```python
from build123d import *

# Parameters (mm, degrees)
SKETCH1_R                = 2
SKETCH1_R_2              = 2.5
BOSS_EXTRUDE1_DEPTH      = 5
BOSS_EXTRUDE2_DEPTH      = 6.5
BOSS_EXTRUDE2_DEPTH_BACK = 1.5
SKETCH2_R                = 2
CUT_EXTRUDE1_DEPTH       = 100
FILLET1_R                = 0.5


with BuildPart() as part:
    # Sketch1 → Boss-Extrude1 (new body)
    with BuildSketch(Plane.XY):
        with BuildLine():
            Line((7, 0), (13.5, 0))
            Line((13.5, 0), (13.5, 12))
            Line((13.5, 12), (5, 12))
            Line((5, 12), (5, 62.5))
            ThreePointArc((5, 62.5), (9.393398312, 73.106601748), (20.000000086, 77.5))
            Line((20.000000086, 77.5), (42.5, 77.5))
            ThreePointArc((42.5, 77.5), (47, 82), (42.5, 86.5))
            Line((42.5, 86.5), (-42.5, 86.5))
            ThreePointArc((-42.5, 86.5), (-47, 82), (-42.5, 77.5))
            Line((-42.5, 77.5), (-20, 77.5))
            ThreePointArc((-20, 77.5), (-9.393398282, 73.106601718), (-5, 62.5))
            Line((-5, 62.5), (-5, 12))
            Line((-5, 12), (-13.5, 12))
            Line((-13.5, 12), (-13.5, 0))
            Line((-13.5, 0), (-7, 0))
            ThreePointArc((-7, 0), (0, 7), (7, 0))
        make_face()
        with Locations((-42.5, 82)):
            Circle(SKETCH1_R, mode=Mode.SUBTRACT)
        with Locations((0, 82)):
            Circle(SKETCH1_R_2, mode=Mode.SUBTRACT)
        with Locations((42.5, 82)):
            Circle(SKETCH1_R, mode=Mode.SUBTRACT)
    extrude(amount=BOSS_EXTRUDE1_DEPTH)

    # Sketch1_3 → Boss-Extrude2 (add, two sides)
    with BuildSketch(Plane.XY) as boss_extrude2_sk:
        with BuildLine():
            Line((5, 12), (5, 4.898979486))
            ThreePointArc((5, 4.898979486), (6.480740698, 2.645751311), (7, 0))
            Line((7, 0), (13.5, 0))
            Line((13.5, 0), (13.5, 12))
            Line((13.5, 12), (5, 12))
        make_face()
        with BuildLine():
            ThreePointArc((-7, 0), (-6.480740698, 2.645751311), (-5, 4.898979486))
            Line((-5, 4.898979486), (-5, 12))
            Line((-5, 12), (-13.5, 12))
            Line((-13.5, 12), (-13.5, 0))
            Line((-13.5, 0), (-7, 0))
        make_face()
        with BuildLine():
            ThreePointArc((-5, 4.898979486), (-2.711747002, 6.453404388), (0, 7))
            Line((0, 7), (0, 12))
            Line((0, 12), (-5, 12))
            Line((-5, 12), (-5, 4.898979486))
        make_face()
        with BuildLine():
            Line((0, 12), (0, 7))
            ThreePointArc((0, 7), (2.711747002, 6.453404388), (5, 4.898979486))
            Line((5, 4.898979486), (5, 12))
            Line((5, 12), (0, 12))
        make_face()
    extrude(amount=BOSS_EXTRUDE2_DEPTH)
    extrude(boss_extrude2_sk.sketch, amount=-BOSS_EXTRUDE2_DEPTH_BACK)

    # Sketch2 → Cut-Extrude1 (cut)
    with BuildSketch(Plane(origin=(0, 12, 0), x_dir=(1, 0, 0), z_dir=(0, 1, 0))):
        with Locations((9.5, -2.5)):
            Circle(SKETCH2_R)
        with Locations((-9.5, -2.5)):
            Circle(SKETCH2_R)
    extrude(amount=-CUT_EXTRUDE1_DEPTH, mode=Mode.SUBTRACT)

    # Fillet1
    fillet1_edges = [part.edges().sort_by_distance(p)[0] for p in [
        (5, 12, 2.5),
        (13.5, 12, 2.5),
        (-13.5, 12, 2.5),
        (-5, 12, 2.5),
    ]]
    fillet(fillet1_edges, radius=FILLET1_R)


solid = part.part
```
Geometry check sheet. Reference: the model listing, model coordinates, mm. A direction names the side the tool comes from. Round coordinates to 2 decimals unless told otherwise and drop trailing zeros. Loops run counter-clockwise (first coordinate to the right, second up) from the corner with the lowest first, then second, coordinate; pieces in that order, holes last. Notation, with made-up numbers: (-32, 66) - (24, 66) arc R26 cw to (24, 94) - close; hole circle Ø1 at (-28.75, 47). An arc over 180 degrees is marked (long way). Write item = value, one per line. Start each with the question number.
1. Section check B-B on y = 82. Enter the section's corners in (x, z), then the cut area to 3 significant figures.
2. Depth check by flat-ended pin: pin 1 (8 mm diameter, centred on x = -11.5, y = 42.5, fed in from +Z); pin 2 (4 mm diameter, centred on y = 3, z = 2.5, fed in from +X); pin 3 (2.5 mm diameter, centred on y = 8.5, z = 2.5, fed in from -X); pin 4 (1 mm diameter, centred on y = 14.5, z = 3.5, fed in from -X). Enter the tip coordinate at first touch or a pass-through.
3. Section check D-D on y = 9.5. Enter the section's corners in (x, z), then the cut area to 3 significant figures.
4. Thickness scan on line 1 (X direction, y = 8.5, z = 2.5); line 2 (Z direction, x = 9.5, y = 5.75); line 3 (Y direction, x = -42.5, z = 3.65). Record the ranges inside material, lowest first.
5. Section check C-C on x = 9.5. Enter the section's corners in (y, z).
6. Set-up check for faces 5 (the face through (0, 63, 5)), 6 (the face through (13.5, 6, 3)), 7 (the face through (7.9, 6.1, 3.7)): record each of +Z, -Z, +X, -X, +Y, -Y from which the full face is reachable in a straight line by a thin tool's end or side.
7. Section check A-A on z = 2.5. Give the number of separate pieces and of enclosed holes in the cut face, then the cut area to 3 significant figures.
8. Mould release check, pull along X, two halves, no side actions. Record for faces 1 (the face through (31, 77.5, 2)), 2 (the face through (5, 37, 2)), 3 (the face through (-11.1, 6.1, 3.7)), 4 (the face through (-9.51, 73.22, 2.46)): released by +X, released by -X, zero draft, split by the parting line, or undercut.
Working result:
q1.outline = (-47, 0) - (-44.5, 0) - (-44.5, 5) - (-47, 5) - close; (-40.5, 0) - (-2.5, 0) - (-2.5, 5) - (-40.5, 5) - close; (2.5, 0) - (40.5, 0) - (40.5, 5) - (2.5, 5) - close; (44.5, 0) - (47, 0) - (47, 5) - (44.5, 5) - close
q1.area = 405 mm^2
q2.pin_1 = through
q2.pin_2 = 13.5
q2.pin_3 = -13.5
q2.pin_4 = -5
q3.outline = (-13.5, -1.5) - (13.5, -1.5) - (13.5, 6.5) - (-13.5, 6.5) - close; hole circle Ø4 at (-9.5, 2.5); hole circle Ø4 at (9.5, 2.5)
q3.area = 191 mm^2
q4.line_1 = -13.5 to -11.5, -7.5 to 7.5, 11.5 to 13.5
q4.line_2 = -1.5 to 0.5, 4.5 to 6.5
q4.line_3 = 77.5 to 80, 84 to 86.5
q5.outline = (0, -1.5) - (12, -1.5) - (12, 0.5) - (0, 0.5) - close; (0, 4.5) - (12, 4.5) - (12, 6.5) - (0, 6.5) - close; (73.21, 0) - (86.5, 0) - (86.5, 5) - (73.21, 5) - close
q6.face_5 = +Z, +X, -X, +Y
q6.face_6 = +Z, -Z, +X, -Y
q6.face_7 = -Y
q7.separate_pieces = 3
q7.enclosed_holes = 3
q7.area = 1,690 mm^2
q8.face_1 = zero draft
q8.face_2 = released by +X
q8.face_3 = undercut
q8.face_4 = released by -X
